from build123d import *

# Parameters (mm, degrees)
SKETCH1_W           = 30
SKETCH1_H           = 45
BOSS_EXTRUDE1_DEPTH = 5
SKETCH2_W           = 30
SKETCH2_H           = 5
BOSS_EXTRUDE2_DEPTH = 100
BOSS_EXTRUDE3_DEPTH = 30
FILLET1_R           = 8
SKETCH4_R           = 2.5
CUT_EXTRUDE1_DEPTH  = 132.785002923
CHAMFER1_SIZE       = 2
SKETCH5_W           = 26
SKETCH5_H           = 25
CUT_EXTRUDE2_DEPTH  = 1
BOSS_EXTRUDE5_DEPTH = 3
CUT_EXTRUDE3_DEPTH  = 129.19281303
SKETCH7_R           = 0.848419625
BOSS_EXTRUDE4_DEPTH = 1
FILLET2_R           = 3


with BuildPart() as part:
    # Sketch1 → Boss-Extrude1 (new body)
    with BuildSketch(Plane(origin=(0, 0, 0), x_dir=(1, 0, 0), z_dir=(0, 1, 0))):
        Rectangle(SKETCH1_W, SKETCH1_H)
    extrude(amount=BOSS_EXTRUDE1_DEPTH)

    # Sketch2 → Boss-Extrude2 (add)
    with BuildSketch(Plane(origin=(0, 5, 0), x_dir=(1, 0, 0), z_dir=(0, 1, 0))):
        Rectangle(SKETCH2_W, SKETCH2_H)
    extrude(amount=BOSS_EXTRUDE2_DEPTH)

    # Sketch3 → Boss-Extrude3 (add)
    with BuildSketch(Plane(origin=(15, 0, 0), x_dir=(0, 0, -1), z_dir=(1, 0, 0))):
        Polygon((-2.5, 105), (-17.5, 130.980762114), (-12.303847577, 133.980762114), (2.5, 108.339745962), (2.5, 105), align=None)
    extrude(amount=-BOSS_EXTRUDE3_DEPTH)

    # Fillet1
    fillet1_edges = [part.edges().sort_by_distance(p)[0] for p in [
        (0, 5, -2.5),
        (0, 5, 2.5),
        (0, 105, 2.5),
        (0, 108.339745962, -2.5),
    ]]
    fillet(fillet1_edges, radius=FILLET1_R)

    # Sketch4 → Cut-Extrude1 (cut, through all)
    with BuildSketch(Plane(origin=(0, 5, 0), x_dir=(1, 0, 0), z_dir=(0, 1, 0))):
        with Locations(Location((0, 16, 0), (0, 0, 270))):
            Circle(SKETCH4_R)
        with Locations(Location((0, -16, 0), (0, 0, 270))):
            Circle(SKETCH4_R)
    extrude(amount=-CUT_EXTRUDE1_DEPTH, mode=Mode.SUBTRACT)

    # Chamfer1
    chamfer1_edges = [part.edges().sort_by_distance(p)[0] for p in [
        (0, 5, -18.5),
        (0, 5, 13.5),
    ]]
    chamfer(chamfer1_edges, length=CHAMFER1_SIZE)

    # Sketch5 → Cut-Extrude2 (cut)
    with BuildSketch(Plane(origin=(0, 28.167468245, -48.787486121), x_dir=(1, 0, 0), z_dir=(0, 0.4999999999999981, -0.8660254037844397))):
        with Locations((0, -108.45061659)):
            Rectangle(SKETCH5_W, SKETCH5_H)
    extrude(amount=-CUT_EXTRUDE2_DEPTH, mode=Mode.SUBTRACT)

    # Sketch8 → Boss-Extrude5 (add)
    with BuildSketch(Plane(origin=(0, 25.167468245, -43.591333699), x_dir=(1, 0, 0), z_dir=(0, -0.49999999999999784, 0.8660254037844399))):
        with BuildLine():
            Line((-9.746794345, 112.45061659), (-7.826237921, 112.45061659))
            ThreePointArc((-7.826237921, 112.45061659), (-10.5, 105.45061659), (-7.826237921, 98.45061659))
            Line((-7.826237921, 98.45061659), (-9.746794345, 98.45061659))
            ThreePointArc((-9.746794345, 98.45061659), (-12, 105.45061659), (-9.746794345, 112.45061659))
        make_face()
        with BuildLine():
            Line((7.826237921, 98.45061659), (9.746794345, 98.45061659))
            ThreePointArc((9.746794345, 98.45061659), (12, 105.45061659), (9.746794345, 112.45061659))
            Line((9.746794345, 112.45061659), (7.826237921, 112.45061659))
            ThreePointArc((7.826237921, 112.45061659), (10.5, 105.45061659), (7.826237921, 98.45061659))
        make_face()
    extrude(amount=BOSS_EXTRUDE5_DEPTH)

    # Sketch6 → Cut-Extrude3 (cut, through all)
    with BuildSketch(Plane(origin=(0, 25.167468245, -43.591333699), x_dir=(1, 0, 0), z_dir=(0, -0.49999999999999784, 0.8660254037844399))):
        Polygon((-5, 100.45061659), (5, 100.45061659), (5, 114.45061659), (10.5, 114.45061659), (10.5, 120.45061659), (-5, 120.45061659), align=None)
    extrude(amount=-CUT_EXTRUDE3_DEPTH, mode=Mode.SUBTRACT)

    # Sketch7 → Boss-Extrude4 (add)
    with BuildSketch(Plane(origin=(0, 27.667468245, -47.921460718), x_dir=(1, 0, 0), z_dir=(0, 0.4999999999999983, -0.8660254037844397))):
        with Locations(Location((10.5, -105.95061659, 0), (0, 0, 270))):
            Circle(SKETCH7_R)
        with Locations(Location((-10.5, -118.45061659, 0), (0, 0, 270))):
            Circle(SKETCH7_R)
    extrude(amount=BOSS_EXTRUDE4_DEPTH)

    # Fillet2
    fillet2_edges = [part.edges().sort_by_distance(p)[0] for p in [
        (12, 116.490381057, 9.133974596),
        (-12, 116.490381057, 9.133974596),
    ]]
    fillet(fillet2_edges, radius=FILLET2_R - 0.0001)  # a hair under: the kernel refuses the full size


solid = part.part
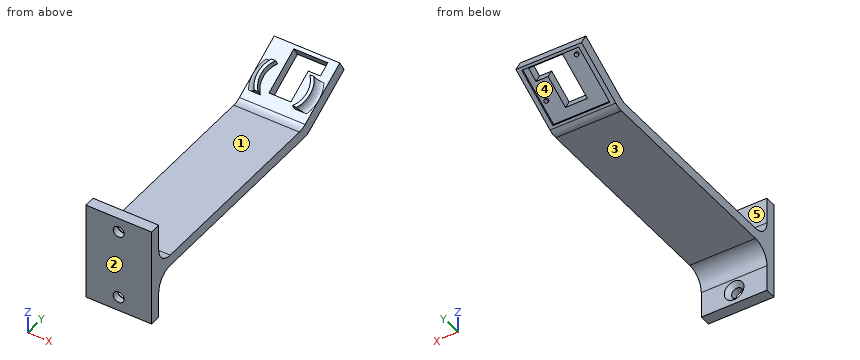
Can you work these out from the model? Positions are in its coordinate system, mm. Face numbers are marked on the shaded views. A direction names the side the tool comes from. Give positions to 0.01 mm unless a question says otherwise; leave off trailing zeros. Loops run counter-clockwise (first coordinate to the right, second up) from the corner with the lowest first, then second, coordinate; pieces in that order, holes last. Notation, with made-up numbers: (11, 7) - (30, 7) arc R23 ccw to (30, 28) - close; hole circle Ø1 at (57, -3). An arc over 180 degrees is marked (long way). One line per item, written item: value.
(1) On a 3-axis mill with a long thin cutter (end or side, diameter ignored), from which of +Z, -Z, +X, -X, +Y, -Y can I reach the whole of each face in a straight line? I mean the marked faces 1, 2 and 3. Say none if no direction works.
Verdict:
face 1: +Z, +X, -X
face 2: +Z, -Z, +X, -X, -Y
face 3: -Z, +X, -X, +Y
(2) I'm going to push flat-ended pins straight in: pin 1 (1 mm diameter, centred on x = 5.5, z = 0, fed in from +Y); pin 2 (3 mm diameter, centred on x = 0, z = -16, fed in from -Y); pin 3 (15 mm diameter, centred on x = 5, y = 68, fed in from -Z); pin 4 (2 mm diameter, centred on x = 5, y = 105, fed in from +Z). Where does each tip first touch, or does it pass through?
Verdict:
pin 1: y = 111.54
pin 2: through
pin 3: z = -2.5
pin 4: z = 3.14
(3) I need wall thicknesses on line 1 along X through (y, z) = (1.05, 16); line 2 along Z through (x, y) = (1.5, 81); line 3 along Y through (x, z) = (-9.5, 4). Which ranges of each line are inside material? Lowest first, please.
Verdict:
line 1: -15 to -2.5, 2.5 to 15
line 2: -2.5 to 2.5
line 3: 0 to 8.34, 107.6 to 117.6
(4) If we section it at C-C, the plane y = 33: List the corners of the cut face in (x, z) for me, plus the area to 3 significant figures.
Verdict:
outline: (-15, -2.5) - (15, -2.5) - (15, 2.5) - (-15, 2.5) - close
area: 150 mm^2
(5) If we section it at A-A, the plane z = -16: List the corners of the cut face in (x, y) for me, plus the area to 3 significant figures.
Verdict:
outline: (-15, 0) - (-2.5, 0) - (-2.5, 3) - (-4.5, 5) - (-15, 5) - close; (2.5, 0) - (15, 0) - (15, 5) - (4.5, 5) - (2.5, 3) - close
area: 121 mm^2
(6) If we section it at B-B, the plane x = 0: State how many separate pieces and enclosed holes the cut face has, plus the area to 3 significant figures.
Verdict:
separate pieces: 4
enclosed holes: 0
area: 757 mm^2
(7) If we mould it in two halves opening along X, with no side actions, what happens to the marked faces 4 and 5? For each: released by +X, released by -X, zero draft, split by the parting line, or undercut.
Verdict:
face 4: undercut
face 5: zero draft
